The model under review builds one solid part; all positions refer to its coordinate system, in mm. Give positions to 0.01 mm unless a question says otherwise; leave off trailing zeros. Loops run counter-clockwise (first coordinate to the right, second up) from the corner with the lowest first, then second, coordinate; pieces in that order, holes last. Notation, with made-up numbers: M 76.5,26.5 L 122.5,26.5 A20 cw 122.5,53.5 Z; hole C 48,-12.5 d2. An arc over 180 degrees is marked long. Put each result on its own line as item: value. Start each with the question number.
```python
from build123d import *

# Parameters (mm, degrees)
SKETCH1_W           = 200
SKETCH1_H           = 250
SKETCH1_W_2         = 5.4862609
SKETCH1_H_2         = 53.998630914
SKETCH1_W_3         = 6.227340135
SKETCH1_H_3         = 10
SKETCH1_W_4         = 9
SKETCH1_H_4         = 6.349855652
SKETCH1_H_5         = 6.350070686
SKETCH1_W_5         = 15
SKETCH1_H_6         = 50
SKETCH1_H_7         = 6.349855651
SKETCH1_W_6         = 10
BOSS_EXTRUDE1_DEPTH = 6.35
FILLET1_R           = 60


with BuildPart() as part:
    # Sketch1 → Boss-Extrude1 (new body)
    with BuildSketch(Plane(origin=(0, 0, 0), x_dir=(1, 0, 0), z_dir=(0, 1, 0))):
        Rectangle(SKETCH1_W, SKETCH1_H)
        with Locations((0, 74.300529772)):
            Rectangle(SKETCH1_W_2, SKETCH1_H_2, mode=Mode.SUBTRACT)
        with Locations((31.053670068, -55)):
            Rectangle(SKETCH1_W_3, SKETCH1_H_3, mode=Mode.SUBTRACT)
        with Locations((31.053670068, -35)):
            Rectangle(SKETCH1_W_3, SKETCH1_H_3, mode=Mode.SUBTRACT)
        with Locations((0, -83.1)):
            Rectangle(SKETCH1_W_4, SKETCH1_H_4, mode=Mode.SUBTRACT)
        with Locations((-31.053670068, -55)):
            Rectangle(SKETCH1_W_3, SKETCH1_H_3, mode=Mode.SUBTRACT)
        with Locations((-31.053670068, -35)):
            Rectangle(SKETCH1_W_3, SKETCH1_H_3, mode=Mode.SUBTRACT)
        with Locations((29, -83.1)):
            Rectangle(SKETCH1_W_4, SKETCH1_H_5, mode=Mode.SUBTRACT)
        with Locations((-84.5, -45)):
            Rectangle(SKETCH1_W_5, SKETCH1_H_6, mode=Mode.SUBTRACT)
        with Locations((-29, -83.1)):
            Rectangle(SKETCH1_W_4, SKETCH1_H_5, mode=Mode.SUBTRACT)
        with Locations((29, -102.149855651)):
            Rectangle(SKETCH1_W_4, SKETCH1_H_5, mode=Mode.SUBTRACT)
        with Locations((0, -102.149855652)):
            Rectangle(SKETCH1_W_4, SKETCH1_H_7, mode=Mode.SUBTRACT)
        with Locations((-29, -102.149855651)):
            Rectangle(SKETCH1_W_4, SKETCH1_H_5, mode=Mode.SUBTRACT)
        with Locations((0, -6.9)):
            Rectangle(SKETCH1_W_4, SKETCH1_H_4, mode=Mode.SUBTRACT)
        with Locations((29, -6.9)):
            Rectangle(SKETCH1_W_4, SKETCH1_H_5, mode=Mode.SUBTRACT)
        with Locations((29, 12.149855651)):
            Rectangle(SKETCH1_W_4, SKETCH1_H_5, mode=Mode.SUBTRACT)
        with Locations((0, 12.149855652)):
            Rectangle(SKETCH1_W_4, SKETCH1_H_7, mode=Mode.SUBTRACT)
        with Locations((-29, 12.149855651)):
            Rectangle(SKETCH1_W_4, SKETCH1_H_5, mode=Mode.SUBTRACT)
        with Locations((-29, -6.9)):
            Rectangle(SKETCH1_W_4, SKETCH1_H_5, mode=Mode.SUBTRACT)
        with Locations((-42, -45)):
            Rectangle(SKETCH1_W_6, SKETCH1_H_6, mode=Mode.SUBTRACT)
        with Locations((84.5, -45)):
            Rectangle(SKETCH1_W_5, SKETCH1_H_6, mode=Mode.SUBTRACT)
        with Locations((42, -45)):
            Rectangle(SKETCH1_W_6, SKETCH1_H_6, mode=Mode.SUBTRACT)
    extrude(amount=BOSS_EXTRUDE1_DEPTH)

    # Fillet1
    fillet1_edges = [part.edges().sort_by_distance(p)[0] for p in [
        (-100, 3.175, -125),
        (100, 3.175, -125),
    ]]
    fillet(fillet1_edges, radius=FILLET1_R)


solid = part.part
```
Item 1: Consider section A-A, the plane z = -52. Write out the cut boundary in (x, y), plus the area to 3 significant figures.
Item 2: Consider section C-C, the plane y = 3.75. Give the number of separate pieces and of enclosed holes in the cut face, plus the area to 3 significant figures.
Item 3: Clearance check with flat-ended pins moving along their axes: pin 1 Ø1.9 at (x, y) = (-42.5, 3) entering from -Z; pin 2 Ø3 at (x, y) = (-81.5, 4) entering from -Z; pin 3 Ø1.9 at (x, y) = (85, 1.5) entering from -Z. State where each tip first meets the part, or that it passes through.
Item 4: To check wall thickness, follow L1, parallel to Z at x = -2, y = 2.25; L2, parallel to X at y = 2.5, z = 61; L3, parallel to Z at x = 26, y = 4.25. State the ranges of each line that lie inside material, in increasing order. Write a range as [from, to].
Item 5: Draft analysis for pull direction Z (two halves, no side actions). For faces 1 (the flat face through (4.5, 3, 102)), 2 (the flat face through (-1, 0, -2)), 3 (the cylindrical face through (81.96, 3.22, -107.89)), state which applies: +Z half, -Z half, draft (parallel to the pull), parting line (faces both ways), or undercut.
Item 6: Consider section B-B, the plane x = -85.5. Write out the cut boundary in (y, z), plus the area to 3 significant figures.
Report:
1. outline: M -100,0 L -2.74,0 L -2.74,6.35 L -100,6.35 Z; M 2.74,0 L 100,0 L 100,6.35 L 2.74,6.35 Z
1. area: 1,240 mm²
2. separate pieces: 1
2. enclosed holes: 21
2. area: 44,700 mm²
3. pin 1: z = -124.98
3. pin 2: z = -109.72
3. pin 3: z = -105.74
4. L1: [-125, -101.3], [-47.3, -15.32], [-8.97, 3.73], [10.07, 79.93], [86.27, 98.97], [105.32, 125]
4. L2: [-100, -92], [-77, -47], [-37, 37], [47, 77], [92, 100]
4. L3: [-125, -15.32], [-8.97, 3.72], [10.08, 79.92], [86.28, 98.97], [105.32, 125]
5. face 1: undercut
5. face 2: draft
5. face 3: -Z half
6. outline: M 0,-104.11 L 6.35,-104.11 L 6.35,20 L 0,20 Z; M 0,70 L 6.35,70 L 6.35,125 L 0,125 Z
6. area: 1,140 mm²
